Check sheet for the modelled part. Datum: model origin and axes. Units: mm. A direction names the side the tool comes from. Coordinates: 2 decimals unless noted, no trailing zeros. Loops run counter-clockwise (first coordinate to the right, second up) from the corner with the lowest first, then second, coordinate; pieces in that order, holes last. Notation, with made-up numbers: M 46.5,48.25 L 61.5,48.25 A14 cw 61.5,52.25 Z; hole C -0.5,-39 d10. An arc over 180 degrees is marked long. Use CSV: the item, a comma, the result in double quotes. Start each with the question number.
(1) Section check B-B on y = 3.5. Record the cut outline in (x, z) (3 decimals).
(2) Set-up check for faces 1 (the cylindrical face through (-17.35, 22.01, -8.47)), 2 (the cylindrical face through (6.586, 10.329, 0.084)), 3 (the flat face through (-9.14, 9.55, 8.59)): record each of +Z, -Z, +X, -X, +Y, -Y from which the full face is reachable in a straight line by a thin tool's end or side.
(3) Section check D-D on x = 0. Record the cut outline in (y, z) (3 decimals), and give its area (3 significant figures).
(4) Section check A-A on z = 0. Record the cut outline in (x, y), and give its area (3 significant figures).
(5) Draft check along Y on faces 4 (the cylindrical face through (-2.262, 1.734, 6.9)), 5 (the cylindrical face through (0, -5, 9)), 6 (the cylindrical face through (-2.262, -1.734, -9.904)), 7 (the flat face through (18.25, 22, 0)). Enter one of: pulls with the +Y half, pulls with the -Y half, needs draft (parallel to the pull), parting line crosses it, or undercut.
(6) Go/stop test with flat-tipped pins: pin 1 Ø1 at (x, y) = (9.5, 11) entering from -Z (3 decimals); pin 2 Ø4 at (x, z) = (3.5, -5) entering from -Y; pin 3 Ø19.5 at (x, y) = (4, 6) entering from +Z; pin 4 Ø4 at (y, z) = (0.5, -6.5) entering from -X. Record where each tip stops, or that it passes through.
(7) Section check C-C on x = -14.5. Record the cut outline in (y, z) (3 decimals), and give its area (3 significant figures).
(8) Scan lines: line 1 (X direction, y = 22.1, z = 0); line 2 (Z direction, x = 14.5, y = 22.3) (3 decimals); line 3 (Z direction, x = -3.5, y = 18) (3 decimals). Record each from-to range of solid material in increasing order.
Autodesk Inventor part; units mm, degrees
ref_plane "YZ Plane" through (0, 0, 0) normal (1, 0, 0) x (0, 1, 0)
ref_plane "XZ Plane" through (0, 0, 0) normal (0, 1, 0) x (-1, 0, 0)
ref_plane "XY Plane" through (0, 0, 0) normal (0, 0, 1) x (1, 0, 0)
sketch "スケッチ1" plane through (0, 0, 0) normal (0, 0, 1) x (1, 0, 0)
  circle A0 centre (0, 0) radius 12.25
  circle A1 centre (0, 0) radius 2.85
  circle A2 centre (0, 0) radius 5
  line L0 (4.6517, -1.8335) -> (13.75, 21.25)
  line L1 (0, 0) -> (0, -12.25) construction
  line L2 (0, 21.25) -> (18.25, 21.25)
  line L3 (18.25, 21.25) -> (18.25, 22.75)
  line L4 (18.25, 22.75) -> (0, 22.75)
  line L5 (0, 22.75) -> (0, 21.25)
  line L6 (-4.6517, -1.8335) -> (-13.75, 21.25)
  line L7 (0, 21.25) -> (-18.25, 21.25)
  line L8 (-18.25, 21.25) -> (-18.25, 22.75)
  line L9 (-18.25, 22.75) -> (0, 22.75)
  dimension "d0" = 24.5
  dimension "d2" = 10
  dimension "d1" = 5.7
  dimension "d4" = 1.5
  dimension "d5" = 4.5
  dimension "d6" = 35
  dimension "d7" = 18.25
extrude "押し出し1" add sketch "スケッチ1" along normal mid plane 12 contours A0 L6 A2 L0 | L0 A2 L6 A0 | A2
extrude "押し出し2" add sketch "スケッチ1" along normal mid plane 21 contours A1
extrude "押し出し3" add sketch "スケッチ1" along normal mid plane 18.65 contours L2 L5 L4 L3 | L7 L8 L9 L5
extrude "押し出し4" add sketch "スケッチ1" against normal blind 1.5 from surface at 9.325 contours L0 A2 L6 A0 | A0 L6 L7 L2 L0 | A2 picked at (-6.2807, 7.4899)
mirror "ミラー1" about plane through (0, 0, 0) normal (0, 0, 1) of "押し出し4"
sketch "スケッチ2" plane through (-18.25, 22.75, -9.325) normal (0, 1, 0) x (1, 0, 0)
  line L0 (36.5, 0) -> (36.5, -18.65)
  line L1 (0, 0) -> (36.5, 0)
  line L2 (0, -18.65) -> (0, 0)
  line L3 (36.5, -18.65) -> (0, -18.65)
  line L4 (0, -9.325) -> (36.5, -9.325)
  line L5 (18.25, 0) -> (18.25, -18.65)
  point P0 (18.25, -9.325)
  point P1 (32.75, -9.325)
  point P2 (3.75, -9.325)
  dimension "d25" = 29
hole "穴1" at (14.5, 22.75, 0) at (-14.5, 22.75, 0) direction (0, -1, 0) diameter 4 end through all
fillet "フィレット1" radius 3 4 edges at (-18.25, 22, -9.325) (-18.25, 22, 9.325) (18.25, 22, 9.325) (18.25, 22, -9.325)
properties part number "caster"
Outcome:
1,outline,"M -11.739,-6 L 11.739,-6 L 11.739,6 L -11.739,6 Z; M -6.754,-9.325 L 6.754,-9.325 L 6.754,-7.825 L -6.754,-7.825 Z; M -6.754,7.825 L 6.754,7.825 L 6.754,9.325 L -6.754,9.325 Z"
2,face 1,"-Z, -X, +Y, -Y"
2,face 2,"none"
2,face 3,"+Z, -X, -Y"
3,outline,"M -12.25,-6 L -2.85,-6 L -2.85,-7.825 L -5,-7.825 L -5,-9.325 L -2.85,-9.325 L -2.85,-10.5 L 2.85,-10.5 L 2.85,-9.325 L 22.75,-9.325 L 22.75,9.325 L 2.85,9.325 L 2.85,10.5 L -2.85,10.5 L -2.85,9.325 L -5,9.325 L -5,7.825 L -2.85,7.825 L -2.85,6 L -12.25,6 Z; hole M 2.85,-7.825 L 21.25,-7.825 L 21.25,7.825 L 2.85,7.825 L 2.85,6 L 12.25,6 L 12.25,-6 L 2.85,-6 Z"
3,area,"435 mm²"
4,outline,"M -18.25,21.25 L -16.5,21.25 L -16.5,22.75 L -18.25,22.75 Z; M -12.5,21.25 L 12.5,21.25 L 12.5,22.75 L -12.5,22.75 Z; C 0,0 d24.5; M 16.5,21.25 L 18.25,21.25 L 18.25,22.75 L 16.5,22.75 Z"
4,area,"514 mm²"
5,face 4,"undercut"
5,face 5,"pulls with the -Y half"
5,face 6,"parting line crosses it"
5,face 7,"needs draft"
6,pin 1,"stops at z = -9.325"
6,pin 2,"stops at y = -12.16"
6,pin 3,"stops at z = 10.5"
6,pin 4,"stops at x = -12.25"
7,outline,"M 21.25,-9.325 L 22.75,-9.325 L 22.75,-2 L 21.25,-2 Z; M 21.25,2 L 22.75,2 L 22.75,9.325 L 21.25,9.325 Z"
7,area,"22.0 mm²"
8,line 1,"x = -18.25 to -16.5, -12.5 to 12.5, 16.5 to 18.25"
8,line 2,"z = -9.325 to -2, 2 to 9.325"
8,line 3,"z = -9.325 to -7.825, 7.825 to 9.325"
